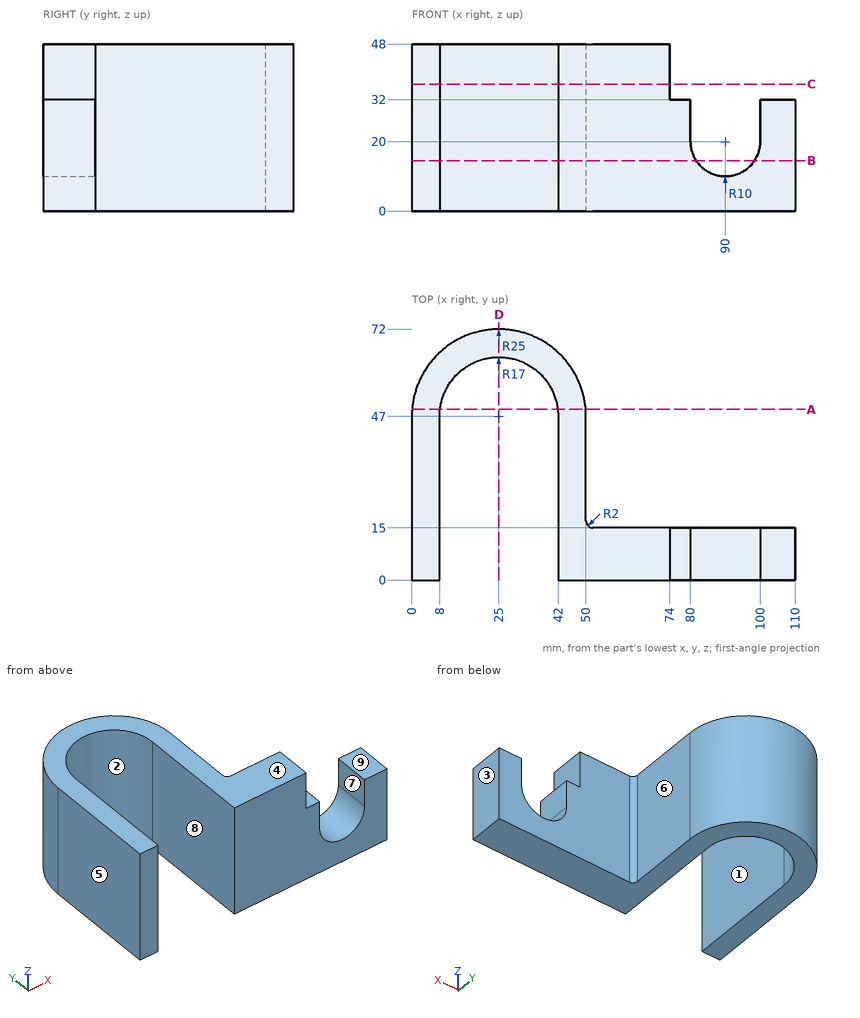
Verification items for this drawing (mm, ordinates from the low corner). A direction names the side the tool comes from. Coordinates: 2 decimals unless noted, no trailing zeros. Write each loop counter-clockwise with the first axis right and the second up, starting at its lowest first coordinate (ties: lowest second). Pieces come first, ordered by that corner, then holes. Notation, with made-up numbers: M -19.75,26.5 L 12.25,26.5 A21 cw 12.25,46.5 Z; hole C -25,-16.5 d7. An arc over 180 degrees is marked long. Use one line per item in the form item = value. Start each with the question number.
1) Section check C-C on z = 36.5. Enter the section's corners in (x, y).
2) Section check B-B on z = 14.5. Enter the section's corners in (x, y).
3) Go/stop test with flat-tipped pins: pin 1 Ø11 at (x, y) = (104, 11) entering from +Z; pin 2 Ø9 at (y, z) = (36.5, 35) entering from +X; pin 3 Ø14.5 at (x, z) = (71.5, 12.5) entering from +Y. Record where each tip stops, or that it passes through.
4) Section check A-A on y = 49. Enter the section's corners in (x, z).
5) Set-up check for the marked faces 5, 6, 7, 8 and 9: record each of +Z, -Z, +X, -X, +Y, -Y from which the full face is reachable in a straight line by a thin tool's end or side.
6) Release check for a two-part mould opening along X. For the marked faces 1, 2, 3 and 4 record: pulls with the +X half, pulls with the -X half, needs draft (parallel to the pull), parting line crosses it, or undercut.
7) Section check D-D on x = 25. Enter the section's corners in (y, z).
8) Thickness scan on probe 1 along X at (y, z) = (46.5, 40.5); probe 2 along X at (y, z) = (3, 7.5); probe 3 along Y at (x, z) = (98.5, 9). Record the ranges inside material, lowest first. Write a range as from..to.
Responses:
q1.outline = M 0,0 L 8,0 L 8,47 A17 cw 42,47 L 42,0 L 74,0 L 74,15 L 52,15 A2 cw 50,17 L 50,47 A25 ccw 0,47 Z
q2.outline = M 0,0 L 8,0 L 8,47 A17 cw 42,47 L 42,0 L 81.65,0 L 81.65,15 L 52,15 A2 cw 50,17 L 50,47 A25 ccw 0,47 Z; M 98.35,0 L 110,0 L 110,15 L 98.35,15 Z
q3.pin_1 = 32
q3.pin_2 = 50
q3.pin_3 = 15
q4.outline = M 0.08,0 L 8.12,0 L 8.12,48 L 0.08,48 Z; M 41.88,0 L 49.92,0 L 49.92,48 L 41.88,48 Z
q5.face_5 = +Z, -Z, -X, +Y, -Y
q5.face_6 = +Z, -Z, +X, +Y
q5.face_7 = +Z, +Y, -Y
q5.face_8 = +Z, -Z, -Y
q5.face_9 = +Z, +X, +Y, -Y
q6.face_1 = undercut
q6.face_2 = undercut
q6.face_3 = pulls with the +X half
q6.face_4 = needs draft
q7.outline = M 64,0 L 72,0 L 72,48 L 64,48 Z
q8.probe_1 = 0..8, 42..50
q8.probe_2 = 0..8, 42..110
q8.probe_3 = 0..15
